from build123d import *

# Parameters (mm, degrees)
BOSS_EXTRUDE1_DEPTH = 10
BOSS_EXTRUDE2_DEPTH = 22
SKETCH3_R           = 1.5
BOSS_EXTRUDE3_DEPTH = 8
SKETCH4_R           = 11
SKETCH4_R_2         = 2.5
BOSS_EXTRUDE4_DEPTH = 2
SKETCH6_R           = 2.5
BOSS_EXTRUDE5_DEPTH = 25


with BuildPart() as part:
    # Sketch1 → Boss-Extrude1 (new body)
    with BuildSketch(Plane(origin=(0, 0, 0), x_dir=(1, 0, 0), z_dir=(0, 1, 0))):
        Polygon((-21, 17), (-17, 21), (17, 21), (21, 17), (21, -17), (17, -21), (-17, -21), (-21, -17), align=None)
    extrude(amount=BOSS_EXTRUDE1_DEPTH)

    # Sketch2 → Boss-Extrude2 (add)
    with BuildSketch(Plane(origin=(0, 10, 0), x_dir=(1, 0, 0), z_dir=(0, 1, 0))):
        with BuildLine():
            Line((-19.335533906, 18.381623382), (-18.381623382, 19.335533906))
            ThreePointArc((-18.381623382, 19.335533906), (-16.759506637, 20.419397663), (-14.846089476, 20.8))
            Line((-14.846089476, 20.8), (14.846089476, 20.8))
            ThreePointArc((14.846089476, 20.8), (16.759506637, 20.419397663), (18.381623382, 19.335533906))
            Line((18.381623382, 19.335533906), (19.335533906, 18.381623382))
            ThreePointArc((19.335533906, 18.381623382), (20.419397663, 16.759506637), (20.8, 14.846089476))
            Line((20.8, 14.846089476), (20.8, -14.846089476))
            ThreePointArc((20.8, -14.846089476), (20.419397663, -16.759506637), (19.335533906, -18.381623382))
            Line((19.335533906, -18.381623382), (18.381623382, -19.335533906))
            ThreePointArc((18.381623382, -19.335533906), (16.759506637, -20.419397663), (14.846089476, -20.8))
            Line((14.846089476, -20.8), (-14.846089476, -20.8))
            ThreePointArc((-14.846089476, -20.8), (-16.759506637, -20.419397663), (-18.381623382, -19.335533906))
            Line((-18.381623382, -19.335533906), (-19.335533906, -18.381623382))
            ThreePointArc((-19.335533906, -18.381623382), (-20.419397663, -16.759506637), (-20.8, -14.846089476))
            Line((-20.8, -14.846089476), (-20.8, 14.846089476))
            ThreePointArc((-20.8, 14.846089476), (-20.419397663, 16.759506637), (-19.335533906, 18.381623382))
        make_face()
    extrude(amount=BOSS_EXTRUDE2_DEPTH)

    # Sketch3 → Boss-Extrude3 (add)
    # profile 1 of 2: a face of its own
    with BuildSketch(Plane(origin=(0, 32, 0), x_dir=(1, 0, 0), z_dir=(0, 1, 0))):
        Polygon((-17, 21), (-21, 17), (-21, -17), (-17, -21), (17, -21), (21, -17), (21, 17), (17, 21), align=None)
        with BuildLine():
            ThreePointArc((-14.846089476, 20.8), (-16.759506637, 20.419397663), (-18.381623382, 19.335533906))
            Line((-18.381623382, 19.335533906), (-19.335533906, 18.381623382))
            ThreePointArc((-19.335533906, 18.381623382), (-20.419397663, 16.759506637), (-20.8, 14.846089476))
            Line((-20.8, 14.846089476), (-20.8, -14.846089476))
            ThreePointArc((-20.8, -14.846089476), (-20.419397663, -16.759506637), (-19.335533906, -18.381623382))
            Line((-19.335533906, -18.381623382), (-18.381623382, -19.335533906))
            ThreePointArc((-18.381623382, -19.335533906), (-16.759506637, -20.419397663), (-14.846089476, -20.8))
            Line((-14.846089476, -20.8), (14.846089476, -20.8))
            ThreePointArc((14.846089476, -20.8), (16.759506637, -20.419397663), (18.381623382, -19.335533906))
            Line((18.381623382, -19.335533906), (19.335533906, -18.381623382))
            ThreePointArc((19.335533906, -18.381623382), (20.419397663, -16.759506637), (20.8, -14.846089476))
            Line((20.8, -14.846089476), (20.8, 14.846089476))
            ThreePointArc((20.8, 14.846089476), (20.419397663, 16.759506637), (19.335533906, 18.381623382))
            Line((19.335533906, 18.381623382), (18.381623382, 19.335533906))
            ThreePointArc((18.381623382, 19.335533906), (16.759506637, 20.419397663), (14.846089476, 20.8))
            Line((14.846089476, 20.8), (-14.846089476, 20.8))
        make_face(mode=Mode.SUBTRACT)
    # profile 2 of 2: a face of its own
    with BuildSketch(Plane(origin=(0, 32, 0), x_dir=(1, 0, 0), z_dir=(0, 1, 0))):
        with BuildLine():
            Line((14.846089476, 20.8), (-14.846089476, 20.8))
            ThreePointArc((-14.846089476, 20.8), (-16.759506637, 20.419397663), (-18.381623382, 19.335533906))
            Line((-18.381623382, 19.335533906), (-19.335533906, 18.381623382))
            ThreePointArc((-19.335533906, 18.381623382), (-20.419397663, 16.759506637), (-20.8, 14.846089476))
            Line((-20.8, 14.846089476), (-20.8, -14.846089476))
            ThreePointArc((-20.8, -14.846089476), (-20.419397663, -16.759506637), (-19.335533906, -18.381623382))
            Line((-19.335533906, -18.381623382), (-18.381623382, -19.335533906))
            ThreePointArc((-18.381623382, -19.335533906), (-16.759506637, -20.419397663), (-14.846089476, -20.8))
            Line((-14.846089476, -20.8), (14.846089476, -20.8))
            ThreePointArc((14.846089476, -20.8), (16.759506637, -20.419397663), (18.381623382, -19.335533906))
            Line((18.381623382, -19.335533906), (19.335533906, -18.381623382))
            ThreePointArc((19.335533906, -18.381623382), (20.419397663, -16.759506637), (20.8, -14.846089476))
            Line((20.8, -14.846089476), (20.8, 14.846089476))
            ThreePointArc((20.8, 14.846089476), (20.419397663, 16.759506637), (19.335533906, 18.381623382))
            Line((19.335533906, 18.381623382), (18.381623382, 19.335533906))
            ThreePointArc((18.381623382, 19.335533906), (16.759506637, 20.419397663), (14.846089476, 20.8))
        make_face()
        with Locations(Location((15.5, 15.5, 0), (0, 0, 270))):
            Circle(SKETCH3_R, mode=Mode.SUBTRACT)
        with Locations(Location((15.5, -15.5, 0), (0, 0, 270))):
            Circle(SKETCH3_R, mode=Mode.SUBTRACT)
        with Locations(Location((-15.5, 15.5, 0), (0, 0, 270))):
            Circle(SKETCH3_R, mode=Mode.SUBTRACT)
        with Locations(Location((-15.5, -15.5, 0), (0, 0, 270))):
            Circle(SKETCH3_R, mode=Mode.SUBTRACT)
    extrude(amount=BOSS_EXTRUDE3_DEPTH)

    # Sketch4 → Boss-Extrude4 (add)
    with BuildSketch(Plane(origin=(0, 40, 0), x_dir=(1, 0, 0), z_dir=(0, 1, 0))):
        with Locations(Location((0, 0, 0), (0, 0, 270))):
            Circle(SKETCH4_R)
        with Locations(Location((0, 0, 0), (0, 0, 270))):
            Circle(SKETCH4_R_2, mode=Mode.SUBTRACT)
    extrude(amount=BOSS_EXTRUDE4_DEPTH)

    # Sketch6 → Boss-Extrude5 (add)
    with BuildSketch(Plane(origin=(0, 40, 0), x_dir=(1, 0, 0), z_dir=(0, 1, 0))):
        with Locations(Location((0, 0, 0), (0, 0, 270))):
            Circle(SKETCH6_R)
    extrude(amount=BOSS_EXTRUDE5_DEPTH)


solid = part.part
Can you work these out from the model? Positions are in its coordinate system, mm. A direction names the side the tool comes from. Coordinates: 2 decimals unless noted, no trailing zeros. Order: outer loops, then holes, each group sorted by start corner. A loop starts at its lowest first (then second) coordinate and runs counter-clockwise, first axis right, second up. Notation, with made-up numbers: (-18.75, 24.25) - (20.25, 24.25) arc R19 cw to (20.25, 45.25) - close; hole circle Ø8 at (19.25, -31.75). An arc over 180 degrees is marked (long way). Answer as a JSON object with one key per item and string values. Group by question number.
Q1. Imagine slicing it at C-C (y = 6). Please give me the cut outline in (x, z), and give its area (3 significant figures).
Q2. Imagine slicing it at B-B (z = 0). Please give me the cut outline in (x, y).
Q3. Will these pins go through, and if not, where does the flat tip stop? P1, Ø2, axis at x = -6.5, z = -8, coming from the +Y side; P2, Ø3.5, axis at x = 15.5, z = -15.5, coming from the +Y side; P3, Ø1.5, axis at y = 24.5, z = -2, coming from the +X side.
Q4. On a 3-axis mill with a long thin cutter (end or side, diameter ignored), from which of +Z, -Z, +X, -X, +Y, -Y can I reach the whole of each face in a straight line? I mean faces 5 (the face through (-19, 5, -19)), 6 (the face through (20.8, 21, 0)), 7 (the face through (-15.43, 35.94, 14)). Say none if no direction works.
Q5. Imagine slicing it at D-D (y = 30). Please give me the cut outline in (x, z), and give its area (3 significant figures).
Q6. We'd pull the mould along Y, two halves only. Please class faces 1 (the face through (-19, 36, 19)), 2 (the face through (20.41, 20.85, -16.78)), 3 (the face through (-16.78, 20.85, -20.41)), 4 (the face through (0, 42, -3)): +Y half, -Y half, draft (parallel to the pull), parting line (faces both ways), or undercut.
Q7. I need wall thicknesses on line 1 (X direction, y = 36.75, z = -15.5); line 2 (X direction, y = 35, z = 15); line 3 (X direction, y = 15, z = 3). Which ranges of each line are inside material? Lowest first, please. Write a range as from..to.
Q8. Imagine slicing it at A-A (x = 0). Please give me the cut outline in (y, z).
Determined:
{
 "1": {"outline": "(-21, -17) - (-17, -21) - (17, -21) - (21, -17) - (21, 17) - (17, 21) - (-17, 21) - (-21, 17) - close", "area": "1,730 mm2"},
 "2": {"outline": "(-21, 0) - (21, 0) - (21, 10) - (20.8, 10) - (20.8, 32) - (21, 32) - (21, 40) - (11, 40) - (11, 42) - (2.5, 42) - (2.5, 65) - (-2.5, 65) - (-2.5, 42) - (-11, 42) - (-11, 40) - (-21, 40) - (-21, 32) - (-20.8, 32) - (-20.8, 10) - (-21, 10) - close"},
 "3": {"P1": "stops at y = 42", "P2": "stops at y = 40", "P3": "stops at x = 20.8"},
 "4": {"face 5": "-Z, -X, +Y, -Y", "face 6": "+Z, -Z, +X", "face 7": "+Y"},
 "5": {"outline": "(-20.8, -14.85) arc R5 ccw to (-19.34, -18.38) - (-18.38, -19.34) arc R5 ccw to (-14.85, -20.8) - (14.85, -20.8) arc R5 ccw to (18.38, -19.34) - (19.34, -18.38) arc R5 ccw to (20.8, -14.85) - (20.8, 14.85) arc R5 ccw to (19.34, 18.38) - (18.38, 19.34) arc R5 ccw to (14.85, 20.8) - (-14.85, 20.8) arc R5 ccw to (-18.38, 19.34) - (-19.34, 18.38) arc R5 ccw to (-20.8, 14.85) - close", "area": "1,700 mm2"},
 "6": {"face 1": "draft", "face 2": "undercut", "face 3": "undercut", "face 4": "+Y half"},
 "7": {"line 1": "x = -21..-17, -14..14, 17..21", "line 2": "x = -21..-16.91, -14.09..14.09, 16.91..21", "line 3": "x = -20.8..20.8"},
 "8": {"outline": "(0, -21) - (10, -21) - (10, -20.8) - (32, -20.8) - (32, -21) - (40, -21) - (40, -11) - (42, -11) - (42, -2.5) - (65, -2.5) - (65, 2.5) - (42, 2.5) - (42, 11) - (40, 11) - (40, 21) - (32, 21) - (32, 20.8) - (10, 20.8) - (10, 21) - (0, 21) - close"}
}
